Read the model definition and answer for the solid it produces. Units are mm, in the model's axes. A direction names the side the tool comes from. Coordinates: 2 decimals unless noted, no trailing zeros. Write each loop counter-clockwise with the first axis right and the second up, starting at its lowest first coordinate (ties: lowest second). Pieces come first, ordered by that corner, then holes.
Item 1: A tool of negligible diameter and unlimited length cuts with its end or side. For faces 5 (the face through (30, 84, -65)), 6 (the face through (30, 1.5, -66)), 7 (the face through (30, 41, 0)), from which of +Z, -Z, +X, -X, +Y, -Y can it reach the whole face along a straight path? Write none if from no direction.
Item 2: Section A-A (y = 47.5) is taken. Give the vertices of the cut face in (x, z).
Item 3: Each of these flat-tipped pins is pushed along its axis until it touches: P1, Ø6, axis at x = 51.5, y = 12, coming from the +Z side; P2, Ø1.6, axis at x = 0.5, z = 16.5, coming from the -Y side; P3, Ø4, axis at x = 51.5, y = 61.5, coming from the -Z side; P4, Ø24.5, axis at y = 22, z = -73, coming from the -X side. Where does it stop, or does it pass through?
Item 4: Section C-C (x = 41) is taken. Give the vertices of the cut face in (y, z).
Item 5: Straight lines are drawn through the part: probe 1 along Y at (x, z) = (37, -83); probe 2 along X at (y, z) = (32, 25); probe 3 along Z at (x, y) = (56, 72.5). For each, find the intervals that lie inside material, in ascending order.
Item 6: Section B-B (z = -117) is taken. Give the vertices of the cut face in (x, y).
Item 7: Determine the mould class of faces 1 (the face through (30, 0, -65)), 2 (the face through (58.5, 43, -66)), 3 (the face through (1.5, 43, 19)), 4 (the face through (29, 82.5, -66)) for opening direction Y: released by +Y, released by -Y, zero draft, split by the parting line, or undercut.
from build123d import *

# Parameters (mm, degrees)
SKETCH1_W           = 84
SKETCH1_H           = 129
BOSS_EXTRUDE1_DEPTH = 60
SHELL1_T            = -1.5
CUT_EXTRUDE1_DEPTH  = 127.5
SKETCH3_W           = 40
SKETCH3_H           = 84
BOSS_EXTRUDE2_DEPTH = 1.5
SKETCH4_W           = 30.5
SKETCH4_H           = 6.2
CUT_EXTRUDE2_DEPTH  = 165.679233664


with BuildPart() as part:
    # Sketch1 → Boss-Extrude1 (new body)
    with BuildSketch(Plane.YZ):
        with Locations((42, -64.5)):
            Rectangle(SKETCH1_W, SKETCH1_H)
    extrude(amount=BOSS_EXTRUDE1_DEPTH)

    # Shell1
    shell1_openings = [part.faces().sort_by_distance(p)[0] for p in [
        (0, 42, -64.5),
    ]]
    offset(amount=SHELL1_T, openings=shell1_openings, kind=Kind.INTERSECTION)

    # Sketch2 → Cut-Extrude1 (cut)
    with BuildSketch(Plane(origin=(0, 0, -129), x_dir=(1, 0, 0), z_dir=(0, 0, -1))):
        Polygon((1.5, -82.5), (58.5, -82.5), (58.5, -1.5), (1.5, -1.5), (0, -1.5), (0, -82.5), align=None)
    extrude(amount=-CUT_EXTRUDE1_DEPTH, mode=Mode.SUBTRACT)

    # Sketch3 → Boss-Extrude2 (add)
    with BuildSketch(Plane.ZY):
        with Locations((18.5, 42)):
            Rectangle(SKETCH3_W, SKETCH3_H)
    extrude(amount=-BOSS_EXTRUDE2_DEPTH)

    # Sketch4 → Cut-Extrude2 (cut, through all)
    with BuildSketch(Plane(origin=(1.5, 0, 0), x_dir=(0, 0, -1), z_dir=(1, 0, 0))):
        with Locations((-19.25, 28.1)):
            Rectangle(SKETCH4_W, SKETCH4_H)
        with Locations((-19.25, 48.1)):
            Rectangle(SKETCH4_W, SKETCH4_H)
    extrude(amount=-CUT_EXTRUDE2_DEPTH, mode=Mode.SUBTRACT)


solid = part.part
Established:
1. face 5: +Z, -Z, +X, -X, +Y
1. face 6: -Z, -X
1. face 7: +Z, +X, +Y, -Y
2. outline: (0, -1.5) - (58.5, -1.5) - (58.5, -129) - (60, -129) - (60, 0) - (1.5, 0) - (1.5, 4) - (0, 4) - close; (0, 34.5) - (1.5, 34.5) - (1.5, 38.5) - (0, 38.5) - close
3. P1: stops at z = 0
3. P2: stops at y = 0
3. P3: stops at z = -1.5
3. P4: stops at x = 58.5
4. outline: (0, -129) - (1.5, -129) - (1.5, -1.5) - (82.5, -1.5) - (82.5, -129) - (84, -129) - (84, 0) - (0, 0) - close
5. probe 1: y = 0 to 1.5, 82.5 to 84
5. probe 2: x = 0 to 1.5
5. probe 3: z = -1.5 to 0
6. outline: (0, 0) - (60, 0) - (60, 84) - (0, 84) - (0, 82.5) - (58.5, 82.5) - (58.5, 1.5) - (0, 1.5) - close
7. face 1: released by -Y
7. face 2: undercut
7. face 3: zero draft
7. face 4: undercut
